Autodesk Inventor part; units mm, degrees
ref_plane "YZ Plane" through (0, 0, 0) normal (1, 0, 0) x (0, 1, 0)
ref_plane "XZ Plane" through (0, 0, 0) normal (0, 1, 0) x (-1, 0, 0)
ref_plane "XY Plane" through (0, 0, 0) normal (0, 0, 1) x (1, 0, 0)
sketch "Sketch1" plane through (0, 0, 0) normal (0, 1, 0) x (-1, 0, 0)
  line L0 (0, 0) -> (5.6922, -5.6922)
  line L1 (0, 0) -> (8.05, 0) construction
  circle A0 centre (5.6922, -5.6922) radius 1.5
  circle A1 centre (5.6922, 5.6922) radius 1.5
  circle A2 centre (-5.6922, 5.6922) radius 1.5
  circle A3 centre (-5.6922, -5.6922) radius 1.5
  circle A4 centre (0, 100) radius 14
  circle A5 centre (0, 100) radius 2
  line L2 (-50, -14) -> (50, -14)
  line L3 (50, -14) -> (50, 14)
  line L4 (50, 14) -> (-50, 14)
  line L5 (-50, 14) -> (-50, -14)
  line L6 (-50, -14) -> (50, 14) construction
  line L7 (50, -14) -> (-50, 14) construction
  circle A6 centre (0, 0) radius 14
  line L8 (-50, 14) -> (-12.9729, 105.2633)
  line L9 (12.9729, 105.2633) -> (50, 14)
  line L10 (10.3153, 90.5346) -> (41.3666, 14)
  line L11 (-10.3153, 90.5346) -> (-41.3666, 14)
  line L12 (0, 86) -> (0, 14)
  circle A7 centre (0, 100) radius 6
  line L13 (-10.3153, 90.5346) -> (-5.5598, 102.2557)
  line L14 (10.3153, 90.5346) -> (5.5598, 102.2557)
  line L15 (-40, 14) -> (-40, -14)
  line L16 (40, 13) -> (40, -14)
  circle A8 centre (0, 0) radius 4
  circle A9 centre (0, 100) radius 70
  circle A10 centre (0, 100) radius 80
  line L17 (-40, 14) -> (-40, 30.718)
  line L18 (-14, 0) -> (-14, 21.2345)
  line L19 (14, 0) -> (14, 21.2345)
  line L20 (40, 13) -> (40, 30.718)
  line L21 (41.3666, 14) -> (40, 12.0487)
  line L22 (-41.3666, 14) -> (-40, 17.3685)
  point P0 (4, 86.5836)
  point P1 (2.5, 14)
  point P2 (-4, 86.5836)
  point P3 (4, 95.5279)
  point P4 (-4, 95.5279)
  point P5 (4.6667, 30.1557)
  point P6 (-4.6667, 30.1557)
  point P7 (31.7797, 37.6297)
  point P8 (-31.7797, 37.6297)
  point P9 (-42.585, 32.2762)
  point P10 (-14, 14)
  point P11 (14, 14)
  point P12 (42.585, 32.2762)
  point P13 (40, 14)
  point P14 (40, 38.6477)
  point P15 (0, 14)
  point P16 (-40, 38.6477)
  point P17 (-40, 17.3685)
  point P18 (-35.5513, 28.3334)
  point P19 (40, 17.3685)
  point P20 (35.5513, 28.3334)
  dimension "d7" = 28
  dimension "d0" = 8.05
  dimension "d1" = 45
  dimension "d2" = 3
  dimension "d5" = 360
  dimension "d9" = 4
  dimension "d10" = 100
  dimension "d11" = 28
  dimension "d12" = 28
  dimension "d13" = 8
  dimension "d14" = 8
  dimension "d20" = 10
  dimension "d22" = 10
  dimension "d24" = 8
  dimension "d26" = 140
  dimension "d29" = 10
  dimension "d30" = 100
extrude "Extrusion1" add sketch "Sketch1" along normal blind 2 contours A4 L14 A7 L13 | A4 L9 A9 L10 | A4 L11 A9 L8 | L9 A10 L10 A9 | L10 A10 L12 A9 | A7 | A9 L11 A10 L8 | L9 L4 L10 L20 A10 | L12 A10 L11 A9 | A10 L20 L10 | A10 L17 L11 L4 L8 | L3 L2 L16 L21 L4 | A10 L19 L4 L12 | L12 L4 L18 A10 | L10 L4 L20 | L11 L17 A10 | L4 L15 L2 L5 | L21 L16 L20 L4 | A6 L18 L4 | L4 L19 A6 | A6 | L17 L4 L11 picked at (9.3983, 95.3801)
fillet "Fillet1" radius 4 6 edges at (5.5598, 1, 102.2557) (-5.5598, 1, 102.2557) (50, 1, 14) (-50, 1, 14) (-31.7797, 1, 37.6297) (31.7797, 1, 37.6297)
fillet "Fillet2" radius 4 6 edges at (14, 1, 21.2345) (-14, 1, 21.2345) (35.5513, 1, 28.3334) (40, 1, 17.3685) (-35.5513, 1, 28.3334) (-40, 1, 17.3685)
fillet "Fillet3" radius 2 4 edges at (-40, 1, -14) (50, 1, -14) (40, 1, -14) (-50, 1, -14)
equation "\"d14\" = d13"
equation "\"d20\" = d22"
properties part number "frame_rotor" material "Aluminum 6061"
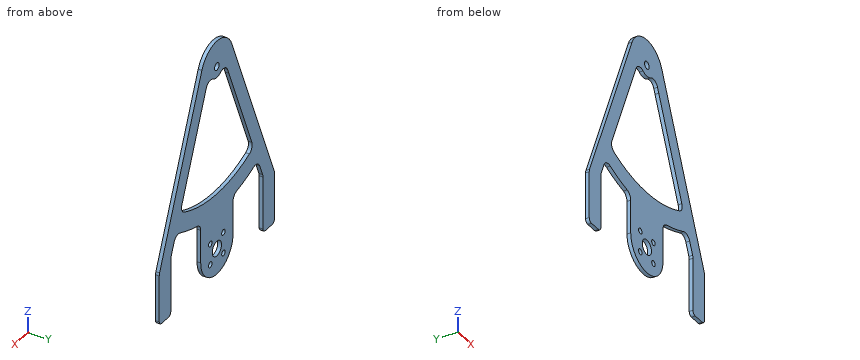
Work out the finished part from the listing and answer in its coordinate system (mm). Coordinates: 2 decimals unless noted, no trailing zeros. Write each loop counter-clockwise with the first axis right and the second up, starting at its lowest first coordinate (ties: lowest second). Pieces come first, ordered by that corner, then holes. Notation, with made-up numbers: M 2,8 L 45,8 A19 ccw 45,15 Z; hole C 70,53 d4. An arc over 180 degrees is marked long. Answer as CSV lines item,"result". Start each with the question number.
Item 1: Flat-ended cylindrical pins translate along their axes: P1, Ø1.8, axis at x = -5.69, z = -5.69, coming from the -Y side; P2, Ø1, axis at x = 9, y = 1, coming from the +Z side; P3, Ø1, axis at y = 1.5, z = 14.5, coming from the -X side. Find the tip coordinate at first contact, or state that the pin passes through.
Item 2: Consider L1, parallel to X at y = 1.5, z = 0; L2, parallel to Z at x = -4.5, y = 0.5; L3, parallel to X at y = 0.7, z = 2. Determine where each line is inside the solid, lowest interval first.
Item 3: Section B-B on z = 72 is taken. Write down the section's boundary in (x, y), and give its area (3 significant figures).
Item 4: Section C-C on x = 26 is taken. Write down the section's boundary in (y, z), and give its area (3 significant figures).
Item 5: Section D-D on z = -2.5 is taken. Write down the section's boundary in (x, y).
Item 6: Section A-A on x = 0 is taken. Write down the section's boundary in (y, z).
Checks:
1,P1,"passes through"
1,P2,"stops at z = 111.12"
1,P3,"stops at x = -49.92"
2,L1,"x = -50 to -40, -14 to -4, 4 to 14, 40 to 50"
2,L2,"z = -13.26 to -6.6, -4.78 to 4.78, 6.6 to 30.14, 95.54 to 113.26"
2,L3,"x = -50 to -40, -14 to -3.46, 3.46 to 14, 40 to 50"
3,outline,"M -26.47,0 L -17.84,0 L -17.84,2 L -26.47,2 Z; M 17.84,0 L 26.47,0 L 26.47,2 L 17.84,2 Z"
3,area,"34.5 mm²"
4,outline,"M 0,24.34 L 2,24.34 L 2,35.01 L 0,35.01 Z; M 0,51.88 L 2,51.88 L 2,73.15 L 0,73.15 Z"
4,area,"63.9 mm²"
5,outline,"M -50,0 L -40,0 L -40,2 L -50,2 Z; M -13.77,0 L -3.12,0 L -3.12,2 L -13.77,2 Z; M 3.12,0 L 13.77,0 L 13.77,2 L 3.12,2 Z; M 40,0 L 50,0 L 50,2 L 40,2 Z"
6,outline,"M 0,-14 L 2,-14 L 2,-4 L 0,-4 Z; M 0,4 L 2,4 L 2,30 L 0,30 Z; M 0,94 L 2,94 L 2,98 L 0,98 Z; M 0,102 L 2,102 L 2,114 L 0,114 Z"
